Work out the finished part from the listing and answer in its coordinate system (mm). A direction names the side the tool comes from. Give positions to 0.01 mm unless a question says otherwise; leave off trailing zeros. Write each loop counter-clockwise with the first axis right and the second up, starting at its lowest first coordinate (ties: lowest second). Pieces come first, ordered by that corner, then holes. Notation, with made-up numbers: (56, 58.5) -> (74, 58.5) arc R14 ccw to (74, 72.5) -> close; hole circle Ø9 at (57, 3). An arc over 180 degrees is marked (long way). Use a Markdown table: item, result. Add a question column.
Q1. Section A-A, the plane y = 0 is taken. Give the vertices of the cut face in (x, z), plus the area to 3 significant figures.
Q2. Section D-D, the plane y = 5.75 is taken. Give the vertices of the cut face in (x, z), plus the area to 3 significant figures.
Q3. Consider line 1 (Y direction, x = -20.5, z = 11); line 2 (Z direction, x = -9, y = 2); line 3 (Y direction, x = -11.5, z = 3). Determine where each line is inside the solid, lowest interval first.
Q4. For faces 1 (the face through (-7.564, -2.13, 5.521)), 2 (the face through (-4.86, -5.53, 36.42)), 3 (the face through (-5, -7, 35.819)), determine the directions among +Z, -Z, +X, -X, +Y, -Y from which every point of the face is accessible in a straight line to the end or side of a thin tool.
Q5. Section B-B, the plane z = 31 is taken. Give the vertices of the cut face in (x, y).
Q6. Each of these flat-tipped pins is pushed along its axis until it touches: pin 1 Ø1.5 at (x, y) = (-15.187, 0) entering from -Z; pin 2 Ø10 at (x, y) = (-11, -2) entering from +Z; pin 3 Ø4 at (x, y) = (8, 7.5) entering from +Z; pin 4 Ø4 at (x, z) = (-4.79, 9.97) entering from +Y. Where does it stop, or does it pass through?
Q7. Section C-C, the plane x = 16 is taken. Give the vertices of the cut face in (y, z), plus the area to 3 significant figures.
Q8. For a pull along Z with two mould halves and no side action, classify faces 4 (the face through (-3, -5, 0)), 5 (the face through (-13, -1.6, 21)), 6 (the face through (-5, -7, 11.819)) as pulls with the +Z half, pulls with the -Z half, needs draft (parallel to the pull), parting line crosses it, or undercut.
from build123d import *

# Parameters (mm, degrees)
SKETCH1_W                 = 43
SKETCH1_H                 = 23
BOSS_EXTRUDE1_DEPTH       = 7
BOSS_EXTRUDE2_DEPTH       = 10
CUT_EXTRUDE1_DEPTH        = 4
M8X1_0_TAPPED_HOLE1_D     = 7
M8X1_0_TAPPED_HOLE1_DEPTH = 3
M8X1_0_TAPPED_HOLE1_TIP   = 2.103012167
M3X0_5_TAPPED_HOLE1_D     = 2.5
SKETCH10_W                = 24
SKETCH10_H                = 12.6
CUT_EXTRUDE2_DEPTH        = 65.606711792
M3X0_5_TAPPED_HOLE2_D     = 2.5
M3X0_5_TAPPED_HOLE2_DEPTH = 7.748924226
M3X0_5_TAPPED_HOLE2_TIP   = 0.751075774
FILLET2_R                 = 10
FILLET3_R                 = 10
FILLET4_R                 = 8.5


with BuildPart() as part:
    # Sketch1 → Boss-Extrude1 (new body)
    with BuildSketch(Plane.XY):
        with Locations((-2.787, -0.099880638)):
            Rectangle(SKETCH1_W, SKETCH1_H)
    extrude(amount=BOSS_EXTRUDE1_DEPTH)

    # Sketch9 → Boss-Extrude2 (add)
    with BuildSketch(Plane(origin=(-10, -11.599880638, 0), x_dir=(0, 0, 1), z_dir=(0, 1, 0))):
        with BuildLine():
            Line((43.646910996, 14.033226444), (35.00321795, 14.033226444))
            ThreePointArc((35.00321795, 14.033226444), (31.483591553, 14.673085952), (28.414378439, 16.510780439))
            ThreePointArc((28.414378439, 16.510780439), (3.5, 5.213), (28.414378439, -6.084780439))
            ThreePointArc((28.414378439, -6.084780439), (31.483591553, -4.247085952), (35.00321795, -3.607226444))
            Line((35.00321795, -3.607226444), (43.646910996, -3.607226444))
            Line((43.646910996, -3.607226444), (43.646910996, 14.033226444))
        make_face()
    extrude(amount=BOSS_EXTRUDE2_DEPTH)

    # Sketch2 → Cut-Extrude1 (cut)
    with BuildSketch(Plane(origin=(0, 0, 0), x_dir=(-1, 0, 0), z_dir=(0, 0, -1))):
        with BuildLine():
            Line((1.32735088, -3.862748758), (4.494142857, -4.089527441))
            ThreePointArc((4.494142857, -4.089527441), (4.787, -4.1), (5.079857143, -4.089527441))
            Line((5.079857143, -4.089527441), (8.24664912, -3.862748758))
            Line((8.24664912, -3.862748758), (20.401285714, -2.992337152))
            ThreePointArc((20.401285714, -2.992337152), (23.187, 0), (20.401285714, 2.992337152))
            Line((20.401285714, 2.992337152), (8.24664912, 3.862748758))
            Line((8.24664912, 3.862748758), (5.079857143, 4.089527441))
            ThreePointArc((5.079857143, 4.089527441), (4.787, 4.1), (4.494142857, 4.089527441))
            Line((4.494142857, 4.089527441), (1.32735088, 3.862748758))
            Line((1.32735088, 3.862748758), (-10.827285714, 2.992337152))
            ThreePointArc((-10.827285714, 2.992337152), (-13.613, 0), (-10.827285714, -2.992337152))
            Line((-10.827285714, -2.992337152), (1.32735088, -3.862748758))
        make_face()
    extrude(amount=-CUT_EXTRUDE1_DEPTH, mode=Mode.SUBTRACT)

    # M8x1.0 Tapped Hole1
    with Locations(Plane(origin=(0, 0, 4), x_dir=(-1, 0, 0), z_dir=(0, 0, -1))):
        with Locations((4.787, 0)):
            Hole(M8X1_0_TAPPED_HOLE1_D / 2, depth=M8X1_0_TAPPED_HOLE1_DEPTH)
            with Locations((0, 0, -(M8X1_0_TAPPED_HOLE1_DEPTH + M8X1_0_TAPPED_HOLE1_TIP / 2))):  # 118° drill point
                Cone(0, M8X1_0_TAPPED_HOLE1_D / 2, M8X1_0_TAPPED_HOLE1_TIP, mode=Mode.SUBTRACT)

    # M3x0.5 Tapped Hole1 (through all)
    with Locations(Plane(origin=(0, 0, 4), x_dir=(-1, 0, 0), z_dir=(0, 0, -1))):
        with Locations((15.187, 0), (-5.613, 0), (4.787, 0)):
            Hole(M3X0_5_TAPPED_HOLE1_D / 2)

    # Sketch10 → Cut-Extrude2 (cut, through all)
    with BuildSketch(Plane(origin=(-23, -11.599880638, 0), x_dir=(0, 0, -1), z_dir=(0, 1, 0))):
        with Locations((-23.818759101, -18.192773556)):
            Rectangle(SKETCH10_W, SKETCH10_H)
    extrude(amount=CUT_EXTRUDE2_DEPTH, mode=Mode.SUBTRACT)

    # M3x0.5 Tapped Hole2
    with Locations(Plane(origin=(-13, -1.599880638, 0), x_dir=(0, 0, -1), z_dir=(0, 1, 0))):
        with Locations((-37.668759101, -8.192773556), (-9.968759101, -8.213)):
            Hole(M3X0_5_TAPPED_HOLE2_D / 2, depth=M3X0_5_TAPPED_HOLE2_DEPTH)
            with Locations((0, 0, -(M3X0_5_TAPPED_HOLE2_DEPTH + M3X0_5_TAPPED_HOLE2_TIP / 2))):  # 118° drill point
                Cone(0, M3X0_5_TAPPED_HOLE2_D / 2, M3X0_5_TAPPED_HOLE2_TIP, mode=Mode.SUBTRACT)

    # Fillet2
    # the kernel refuses this fillet: 10 mm, written as the material it adds along each edge
    with BuildSketch(Plane(origin=(4.850495199, -1.599880638, 7), x_dir=(1, 0, 0), z_dir=(0, -1, 0))) as fillet2_piece_1:
        with BuildLine():
            CenterArc((15.328319752, 9.891985975), FILLET2_R, 176.271875941, 85.299253253)
            Line((5.349481533, 10.542207323), (5.149904768, 10.55521175))
            ThreePointArc((5.149904768, 10.55521175), (3.577273835, 4.813127088), (-0.128339434, 0.153391622))
            Line((-0.128339434, 0.153391622), (0, -0.2))
            ThreePointArc((0, -0.2), (6.931252401, -0.2), (13.833188502, -0.19783972))
            Line((13.833188502, -0.19783972), (13.862504801, 0))
        make_face()
    extrude(amount=10)
    with BuildSketch(Plane(origin=(-14.424495199, -1.599880638, 7), x_dir=(-1, 0, 0), z_dir=(0, -1, 0))) as fillet2_piece_2:
        with BuildLine():
            CenterArc((15.193634372, -8.460440739), FILLET2_R, 122.216027092, 64.805428204)
            Line((5.26862991, -9.682850831), (5.070129821, -9.707299033))
            ThreePointArc((5.070129821, -9.707299033), (3.379125123, -4.436159529), (-0.128339434, -0.153391622))
            Line((-0.128339434, -0.153391622), (0, 0.2))
            ThreePointArc((0, 0.2), (4.931252401, 0.2), (9.75588221, 0.169208815))
            Line((9.75588221, 0.169208815), (9.862504801, 0))
        make_face()
    extrude(amount=10)

    # Fillet3
    # the kernel refuses this fillet: 10 mm, written as the material it takes off along each edge
    with BuildSketch(Plane(origin=(-13.607226444, -36.484775111, 43.646910996), x_dir=(1, 0, 0), z_dir=(0, 1, 0))) as fillet3_piece_1:
        with BuildLine():
            CenterArc((9.953957789, 10), FILLET3_R, 183.8885176, 86.1114824)
            Line((-0.023021105, 9.321846523), (-1.020718995, 9.254031175))
            ThreePointArc((-1.020718995, 9.254031175), (-1, 8.643693046), (-1, 0))
            Line((-1, 0), (0, -1))
            Line((0, -1), (9.953957789, -1))
            Line((9.953957789, -1), (9.953957789, 0))
        make_face()
    extrude(amount=59.769788945, mode=Mode.SUBTRACT)
    with BuildSketch(Plane(origin=(4.033226444, -36.484775111, 43.646910996), x_dir=(0.0024695788781197194, 0, -0.9999969505854329), z_dir=(0, 1, 0))) as fillet3_piece_2:
        with BuildLine():
            CenterArc((9.975387422, 9.978623224), FILLET3_R, 180.141496591, 86.1114824)
            Line((-0.024582084, 9.953927435), (-1.024579034, 9.951457856))
            Line((-1.024579034, 9.951457856), (-0.999996951, -0.002469579))
            Line((-0.999996951, -0.002469579), (0.002469579, -0.999996951))
            ThreePointArc((0.002469579, -0.999996951), (8.646136267, -0.978650669), (9.256523702, -0.997862322))
            Line((9.256523702, -0.997862322), (9.321874949, 0))
        make_face()
    extrude(amount=59.769788945, mode=Mode.SUBTRACT)

    # Fillet4
    fillet4_edges = [part.edges().sort_by_distance(p)[0] for p in [
        (-4.787, -6.599880638, 43.582435806),
    ]]
    fillet(fillet4_edges, radius=FILLET4_R)


solid = part.part
Result set:
| question | item | result |
|---|---|---|
| 1 | outline | (-24.29, 0) -> (-23.19, 0) -> (-23.19, 4) -> (-16.44, 4) -> (-16.44, 7) -> (-24.29, 7) -> close; (-13.94, 4) -> (-8.29, 4) -> (-8.29, 7) -> (-13.94, 7) -> close; (-1.29, 4) -> (4.36, 4) -> (4.36, 7) -> (-1.29, 7) -> close; (6.86, 4) -> (13.61, 4) -> (13.61, 0) -> (18.71, 0) -> (18.71, 7) -> (6.86, 7) -> close |
| 1 | area | 118 mm2 |
| 2 | outline | (-24.29, 0) -> (18.71, 0) -> (18.71, 7) -> (-24.29, 7) -> close |
| 2 | area | 301 mm2 |
| 3 | line 1 | y = -11.6 to -1.6 |
| 3 | line 2 | z = 4 to 7 |
| 3 | line 3 | y = -11.6 to -3.63, 3.63 to 11.4 |
| 4 | face 1 | -Z |
| 4 | face 2 | +Y |
| 4 | face 3 | +Y, -Y |
| 5 | outline | (-14.44, -11.6) -> (-11.11, -11.6) -> (-11.11, -1.6) -> (-14.44, -1.6) -> close; (1.49, -11.6) -> (4.87, -11.6) -> (4.87, -1.6) -> (1.49, -1.6) -> close |
| 6 | pin 1 | passes through |
| 6 | pin 2 | stops at z = 43.04 |
| 6 | pin 3 | stops at z = 7 |
| 6 | pin 4 | stops at y = -1.6 |
| 7 | outline | (-11.6, 0) -> (11.4, 0) -> (11.4, 7) -> (-1.6, 7) -> (-1.6, 7.81) -> (-11.6, 7.81) -> close |
| 7 | area | 169 mm2 |
| 8 | face 4 | pulls with the -Z half |
| 8 | face 5 | needs draft |
| 8 | face 6 | undercut |
